from build123d import *

# Parameters (mm, degrees)
F0_R      = 1.5
F1_DEPTH  = 62.3
F2_R      = 1.5
F3_DEPTH  = 28.3
F5_ANGLE  = 90
F12_R     = 1.5
F13_DEPTH = 70


with BuildPart() as f1:
    # F0 (on Right) → F1 (new body)
    with BuildSketch(Plane.YZ):
        with Locations((0, -40)):
            Circle(F0_R)
    extrude(amount=F1_DEPTH)

    # F2 (on Front) → F3 (join)
    with BuildSketch(Plane.XZ):
        with Locations((0, -40)):
            Circle(F2_R)
    extrude(amount=-F3_DEPTH)

    # F4 (on face) → F5 (revolve)
    with BuildSketch(Plane(origin=(0, 0, 0), x_dir=(0, -1, 0), z_dir=(-1, 0, 0))):
        with BuildLine():
            Line((0, -38.5), (0, -41.5))
            ThreePointArc((0, -41.5), (1.5, -40), (0, -38.5))
        make_face()
    revolve(axis=Axis((0, 0, -40), (0, 0, -1)), revolution_arc=F5_ANGLE)

    # F12 (on face) → F13 (join)
    with BuildSketch(Plane(origin=(2.779995, 1.983642, -39.706263), x_dir=(0.997564, -0.003481, 0.06967), z_dir=(-0.069756, -0.049774, 0.996322))):
        with Locations((-2.786783, -1.995828)):
            Circle(F12_R)
    extrude(amount=F13_DEPTH)


solid = f1.part
The listing builds one solid part. Answer for the finished solid, in the listing's coordinates (mm). A direction names the side the tool comes from. Give positions to 0.01 mm unless a question says otherwise; leave off trailing zeros. Order: outer loops, then holes, each group sorted by start corner. A loop starts at its lowest first (then second) coordinate and runs counter-clockwise, first axis right, second up. Notation, with made-up numbers: (73, -11.75) -> (91, -11.75) arc R18 ccw to (91, -4.75) -> close; hole circle Ø7 at (-13, 44.25). An arc over 180 degrees is marked (long way). Put each result on its own line as item: value.
Item 1: For faces 1 (the face through (62.3, 0, -40)), 2 (the face through (30.714, -0.325, -41.464)), 3 (the face through (-1.2, 14, -40.9)), determine the directions among +Z, -Z, +X, -X, +Y, -Y from which every point of the face is accessible in a straight line to the end or side of a thin tool.
Established:
face 1: +Z, -Z, +X, +Y, -Y
face 2: +X
face 3: +Y
Item 2: A cutting plane is placed at A-A on y = 26.5. Give the vertices of the cut face in (x, z).
Established:
outline: circle Ø3 at (0, -40)
Item 3: Straight lines are drawn through the part: line 1 (Z direction, x = 22.5, y = 1); line 2 (X direction, y = -3, z = -7). For each, find the intervals that lie inside material, in ascending order.
Established:
line 1: z = -41.12 to -38.88
line 2: x = -2.97 to -1.66
